from build123d import *

# Parameters (mm, degrees)
F0_W     = 192.3
F0_H     = 60
F1_DEPTH = 20
F2_W     = 20
F2_H     = 20
F3_DEPTH = 250


with BuildPart() as f1:
    # F0 (on Front) → F1 (new body)
    with BuildSketch(Plane.XZ):
        Rectangle(F0_W, F0_H)
    extrude(amount=F1_DEPTH)

    # F2 (on face) → F3 (join)
    with BuildSketch(Plane(origin=(0, 0, 0), x_dir=(-1, 0, 0), z_dir=(0, 1, 0))):
        with Locations((-86.15, 20)):
            Rectangle(F2_W, F2_H)
        with Locations((86.15, 20)):
            Rectangle(F2_W, F2_H)
    extrude(amount=F3_DEPTH)


solid = f1.part
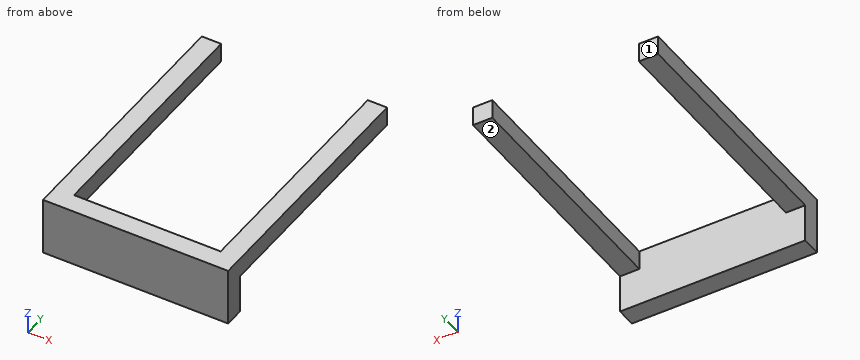
Design review of the part built by this model. Coordinates are the model's own, in mm. Face numbers are marked on the shaded views. A direction names the side the tool comes from. Round coordinates to 2 decimals unless told otherwise and drop trailing zeros. Write each loop counter-clockwise with the first axis right and the second up, starting at its lowest first coordinate (ties: lowest second). Pieces come first, ordered by that corner, then holes. Notation, with made-up numbers: (3, -22) - (41, -22) arc R28 ccw to (41, 15) - close; hole circle Ø11 at (67, -20). An arc over 180 degrees is marked (long way). Return JSON: item names as keys, results as strings. Group by question number.
Item 1: Insertion check: P1, Ø16, axis at x = 85.5, y = 114.5, coming from the -Z side; P2, Ø2, axis at x = -75.5, z = -5.5, coming from the +Y side. Each pin has a flat end and moves straight along its axis. Give the tip position at first contact, or say it passes through.
Item 2: Machinability: for the marked faces 1 and 2, which of the approach directions +Z, -Z, +X, -X, +Y, -Y give a long, thin tool a straight path to every point of the face, cutting with its end or side? Answer none if there is none.
Item 3: We need section D-D on x = -45. Write out the cut boundary in (y, z).
Item 4: We need section A-A on y = 123.5. Write out the cut boundary in (x, z).
Item 5: We need section C-C on x = 82.5. Write out the cut boundary in (y, z).
Item 6: We need section B-B on z = 24.5. Write out the cut boundary in (x, y).
Item 7: For probe 1 along X at (y, z) = (146, 17); probe 2 along Y at (x, z) = (-28, -27); probe 3 along Z at (x, y) = (-88, 94.5), list the stretches that pass through material, from the lowest coordinate up. Write a range as [from, to].
Model answer:
{
 "1": {"P1": "stops at z = 10", "P2": "stops at y = 0"},
 "2": {"face 1": "+Z, -Z, +X, -X, +Y", "face 2": "-Z, +X, -X, +Y"},
 "3": {"outline": "(-20, -30) - (0, -30) - (0, 30) - (-20, 30) - close"},
 "4": {"outline": "(-96.15, 10) - (-76.15, 10) - (-76.15, 30) - (-96.15, 30) - close; (76.15, 10) - (96.15, 10) - (96.15, 30) - (76.15, 30) - close"},
 "5": {"outline": "(-20, -30) - (0, -30) - (0, 10) - (250, 10) - (250, 30) - (-20, 30) - close"},
 "6": {"outline": "(-96.15, -20) - (96.15, -20) - (96.15, 250) - (76.15, 250) - (76.15, 0) - (-76.15, 0) - (-76.15, 250) - (-96.15, 250) - close"},
 "7": {"probe 1": "x = [-96.15, -76.15], [76.15, 96.15]", "probe 2": "y = [-20, 0]", "probe 3": "z = [10, 30]"}
}
